```python
from build123d import *

# Parameters (mm, degrees)
SKETCH1_R           = 9.5
SKETCH1_R_2         = 6
BOSS_EXTRUDE1_DEPTH = 0.5
FILLET1_R           = 0.2


with BuildPart() as part:
    # Sketch1 → Boss-Extrude1 (new body)
    with BuildSketch(Plane(origin=(0, 0, 0), x_dir=(1, 0, 0), z_dir=(0, 1, 0))):
        Circle(SKETCH1_R)
        Circle(SKETCH1_R_2, mode=Mode.SUBTRACT)
    extrude(amount=BOSS_EXTRUDE1_DEPTH)

    # Fillet1
    fillet1_edges = [part.edges().sort_by_distance(p)[0] for p in [
        (-9.5, 0, 0),
        (-9.5, 0.5, 0),
        (-6, 0, 0),
        (-6, 0.5, 0),
    ]]
    fillet(fillet1_edges, radius=FILLET1_R)


solid = part.part
```
The model under review builds one solid part; all positions refer to its coordinate system, in mm. Round coordinates to 2 decimals unless told otherwise and drop trailing zeros. Loops run counter-clockwise (first coordinate to the right, second up) from the corner with the lowest first, then second, coordinate; pieces in that order, holes last. Notation, with made-up numbers: (-39.5, 35.5) -> (-3.5, 35.5) arc R23 ccw to (-3.5, 46.5) -> close; hole circle Ø6 at (-11, -26). An arc over 180 degrees is marked (long way). Answer in a Markdown table with one row per item.
1) Consider section B-B, the plane x = 0. Write out the cut boundary in (y, z).
Taken from the geometry:
| item | result |
|---|---|
| outline | (0, -9.3) arc R0.2 ccw to (0.2, -9.5) -> (0.3, -9.5) arc R0.2 ccw to (0.5, -9.3) -> (0.5, -6.2) arc R0.2 ccw to (0.3, -6) -> (0.2, -6) arc R0.2 ccw to (0, -6.2) -> close; (0, 6.2) arc R0.2 ccw to (0.2, 6) -> (0.3, 6) arc R0.2 ccw to (0.5, 6.2) -> (0.5, 9.3) arc R0.2 ccw to (0.3, 9.5) -> (0.2, 9.5) arc R0.2 ccw to (0, 9.3) -> close |
2) Wall thickness on line 1 along Z through (x, y) = (0, 0.3); line 2 along X through (y, z) = (0.25, -3.75): over which ranges is each line inside the solid? List them lowest first.
Taken from the geometry:
| item | result |
|---|---|
| line 1 | z = -9.5 to -6, 6 to 9.5 |
| line 2 | x = -8.73 to -4.68, 4.68 to 8.73 |
3) Consider section A-A, the plane z = 0. Write out the cut boundary in (x, y).
Taken from the geometry:
| item | result |
|---|---|
| outline | (-9.5, 0.2) arc R0.2 ccw to (-9.3, 0) -> (-6.2, 0) arc R0.2 ccw to (-6, 0.2) -> (-6, 0.3) arc R0.2 ccw to (-6.2, 0.5) -> (-9.3, 0.5) arc R0.2 ccw to (-9.5, 0.3) -> close; (6, 0.2) arc R0.2 ccw to (6.2, 0) -> (9.3, 0) arc R0.2 ccw to (9.5, 0.2) -> (9.5, 0.3) arc R0.2 ccw to (9.3, 0.5) -> (6.2, 0.5) arc R0.2 ccw to (6, 0.3) -> close |
4) For pin 1 Ø2 at (x, z) = (-1.5, 3) entering from -Y, flat-tipped, find the tip position at first contact; note if it passes through.
Taken from the geometry:
| item | result |
|---|---|
| pin 1 | passes through |
